Can you work these out from the model? Positions are in its coordinate system, mm. A direction names the side the tool comes from. Coordinates: 2 decimals unless noted, no trailing zeros. Order: outer loops, then holes, each group sorted by start corner. A loop starts at its lowest first (then second) coordinate and runs counter-clockwise, first axis right, second up. Notation, with made-up numbers: (-6, -1.75) -> (51, -1.75) arc R21 ccw to (51, 12.25) -> close; hole circle Ø2 at (68.5, -37.75). An arc over 180 degrees is marked (long way). Answer in a Markdown table with one row per item.
```python
from build123d import *

# Parameters (mm, degrees)
SKETCH1_W           = 65
SKETCH1_H           = 30
BOSS_EXTRUDE1_DEPTH = 25
SKETCH2_W           = 6.5
SKETCH2_H           = 6.8
CUT_EXTRUDE1_DEPTH  = 31
SKETCH5_R           = 1.5
CUT_EXTRUDE3_DEPTH  = 26
SKETCH6_W           = 6.9
SKETCH6_H           = 6.5
CUT_EXTRUDE4_DEPTH  = 66
SKETCH7_R           = 1.5
CUT_EXTRUDE5_DEPTH  = 10


with BuildPart() as part:
    # Sketch1 → Boss-Extrude1 (new body)
    with BuildSketch(Plane.XY):
        with Locations((28.266423358, -11.605839416)):
            Rectangle(SKETCH1_W, SKETCH1_H)
    extrude(amount=BOSS_EXTRUDE1_DEPTH)

    # Sketch2 → Cut-Extrude1 (cut, through all)
    with BuildSketch(Plane(origin=(0, 3.394160584, 0), x_dir=(1, 0, 0), z_dir=(0, 1, 0))):
        with Locations((57.516423358, -12.9)):
            Rectangle(SKETCH2_W, SKETCH2_H)
        Polygon((54.266423358, -20.6), (54.266423358, -16.3), (54.266423358, -9.5), (54.266423358, -5.2), (46.466423358, -5.2), (46.466423358, -20.6), align=None)
    extrude(amount=-CUT_EXTRUDE1_DEPTH, mode=Mode.SUBTRACT)

    # Sketch5 → Cut-Extrude3 (cut, through all)
    with BuildSketch(Plane.XY.offset(25)):
        with Locations((50.766423358, -2.605839416)):
            Circle(SKETCH5_R)
        with Locations((50.766423358, -9.605839416)):
            Circle(SKETCH5_R)
        with Locations((50.766423358, -16.605839416)):
            Circle(SKETCH5_R)
        with Locations((50.766423358, -23.605839416)):
            Circle(SKETCH5_R)
    extrude(amount=-CUT_EXTRUDE3_DEPTH, mode=Mode.SUBTRACT)

    # Sketch6 → Cut-Extrude4 (cut, through all)
    with BuildSketch(Plane.ZY.offset(4.233576642)):
        Polygon((16.3, -3.105839416), (9.4, -3.105839416), (4.9, -3.105839416), (4.9, -11.405839416), (20.6, -11.405839416), (20.6, -3.105839416), align=None)
        with Locations((12.85, 0.144160584)):
            Rectangle(SKETCH6_W, SKETCH6_H)
    extrude(amount=-CUT_EXTRUDE4_DEPTH, mode=Mode.SUBTRACT)

    # Sketch7 → Cut-Extrude5 (cut)
    with BuildSketch(Plane(origin=(0, 0, 0), x_dir=(-1, 0, 0), z_dir=(0, 0, -1))):
        with Locations((-2.506646914, -6.605839416)):
            Circle(SKETCH7_R)
        with Locations((-15.4668355, -6.605839416)):
            Circle(SKETCH7_R)
        with Locations((-26.853051517, -6.605839416)):
            Circle(SKETCH7_R)
        with Locations((-37.836637843, -6.605839416)):
            Circle(SKETCH7_R)
    extrude(amount=-CUT_EXTRUDE5_DEPTH, mode=Mode.SUBTRACT)


solid = part.part
```
(1) Suppose I cut it at B-B (y = 1.5). Please give me the cut outline in (x, z), and give its area (3 significant figures).
Response values:
| item | result |
|---|---|
| outline | (-4.23, 0) -> (60.77, 0) -> (60.77, 9.4) -> (54.27, 9.4) -> (54.27, 5.2) -> (46.47, 5.2) -> (46.47, 9.4) -> (-4.23, 9.4) -> close; (-4.23, 16.3) -> (46.47, 16.3) -> (46.47, 20.6) -> (54.27, 20.6) -> (54.27, 16.3) -> (60.77, 16.3) -> (60.77, 25) -> (-4.23, 25) -> close |
| area | 1,110 mm2 |
(2) Suppose I cut it at A-A (z = 17.5). Please give me the cut outline in (x, y), and give its area (3 significant figures).
Response values:
| item | result |
|---|---|
| outline | (-4.23, -26.61) -> (46.47, -26.61) -> (46.47, -11.41) -> (-4.23, -11.41) -> close; (-4.23, -3.11) -> (46.47, -3.11) -> (46.47, 3.39) -> (-4.23, 3.39) -> close; (54.27, -26.61) -> (60.77, -26.61) -> (60.77, -11.41) -> (54.27, -11.41) -> close; (54.27, -3.11) -> (60.77, -3.11) -> (60.77, 3.39) -> (54.27, 3.39) -> close |
| area | 1,240 mm2 |
(3) On a 3-axis mill with a long thin cutter (end or side, diameter ignored), from which of +Z, -Z, +X, -X, +Y, -Y can I reach the whole of each face in a straight line? I mean faces 1 (the flat face through (57, 0, 9.4)), 2 (the flat face through (57, -3.106, 7)), 3 (the cylindrical face through (14.08, -7.18, 2.42)). Say none if no direction works.
Response values:
| item | result |
|---|---|
| face 1 | +X, -X, +Y |
| face 2 | +X, -X |
| face 3 | -Z |
(4) We'd pull the mould along X, two halves only. Please class faces 4 (the flat face through (57, -11.406, 18)), 5 (the cylindrical face through (49.268, -23.54, 2.636)), 6 (the flat face through (-4.234, -15, 12)): +X half, -X half, draft (parallel to the pull), parting line (faces both ways), or undercut.
Response values:
| item | result |
|---|---|
| face 4 | draft |
| face 5 | undercut |
| face 6 | -X half |
(5) I need wall thicknesses on line 1 (Z direction, x = 51, y = -18.5); line 2 (Y direction, x = 1, z = 8.75); line 3 (Z direction, x = 21, y = -6.5). Which ranges of each line are inside material? Lowest first, please. Write a range as [from, to].
Response values:
| item | result |
|---|---|
| line 1 | [0, 5.2], [20.6, 25] |
| line 2 | [-26.61, -11.41], [-3.11, 3.39] |
| line 3 | [0, 4.9], [20.6, 25] |
(6) Suppose I cut it at C-C (x = 45). Please give me the cut outline in (y, z).
Response values:
| item | result |
|---|---|
| outline | (-26.61, 0) -> (3.39, 0) -> (3.39, 9.4) -> (-3.11, 9.4) -> (-3.11, 4.9) -> (-11.41, 4.9) -> (-11.41, 20.6) -> (-3.11, 20.6) -> (-3.11, 16.3) -> (3.39, 16.3) -> (3.39, 25) -> (-26.61, 25) -> close |
(7) Suppose I cut it at D-D (z = 4). Count the separate pieces of the cut face and the enclosed holes in it, and give its area (3 significant figures).
Response values:
| item | result |
|---|---|
| separate pieces | 1 |
| enclosed holes | 8 |
| area | 1,890 mm2 |
